Build history of the part. All positions in model axes, mm. Face numbers are marked on the shaded views. A direction names the side the tool comes from. Give positions to 0.01 mm unless a question says otherwise; leave off trailing zeros. Order: outer loops, then holes, each group sorted by start corner. A loop starts at its lowest first (then second) coordinate and runs counter-clockwise, first axis right, second up. Notation, with made-up numbers: M 76.5,4 L 108.5,4 A9 cw 108.5,18 Z; hole C 54,-39.75 d3. An arc over 180 degrees is marked long. One line per item, written item: value.
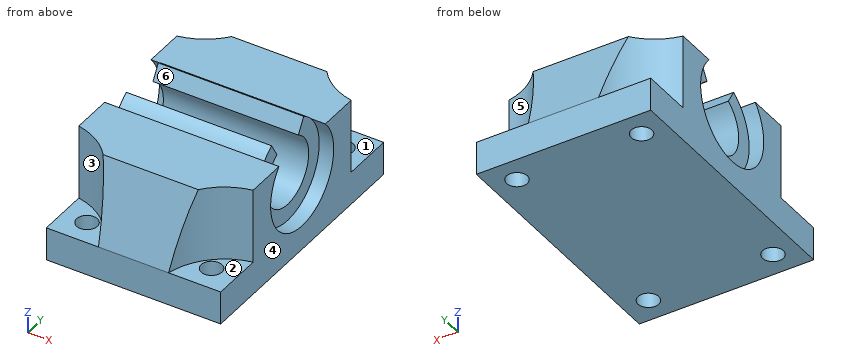
from build123d import *

# Parameters (mm, degrees)
F1_DEPTH = 21
F3_R     = 15.743514377
F4_DEPTH = 33
F5_DEPTH = 17.5
F7_D     = 5


with BuildPart() as f1:
    # F0 (on Right) → F1 (new body, symmetric)
    with BuildSketch(Plane.YZ):
        with BuildLine():
            Line((24.4485357832, 8.14), (8.8170516614, 8.14))
            ThreePointArc((8.8170516614, 8.14), (0, -12), (-8.8170516614, 8.14))
            Line((-8.8170516614, 8.14), (-24.4485357832, 8.14))
            Line((-24.4485357832, 8.14), (-31, -9.86))
            Line((-31, -9.86), (-31, -17.86))
            Line((-31, -17.86), (0, -17.86))
            Line((0, -17.86), (31, -17.86))
            Line((31, -17.86), (31, -9.86))
            Line((31, -9.86), (24.4485357832, 8.14))
        make_face()
    extrude(amount=F1_DEPTH, both=True)

    # F3 (on offset) → F4 (cut)
    with BuildSketch(Plane(origin=(0, 0, -9.86), x_dir=(1, 0, 0), z_dir=(0, 0, -1))):
        with Locations((-23.8725915551, 34.129627049)):
            Circle(F3_R)
        with Locations((-23.8725915551, -34.129627049)):
            Circle(F3_R)
        with Locations((23.8725915551, -34.129627049)):
            Circle(F3_R)
        with Locations((23.8725915551, 34.129627049)):
            Circle(F3_R)
    extrude(amount=-F4_DEPTH, mode=Mode.SUBTRACT)

    # F0 (on Right) → F5 (join, symmetric)
    with BuildSketch(Plane.YZ):
        with BuildLine():
            ThreePointArc((4.0603069037, 6.8930332835), (6.9455905159, 3.9697320294), (8, 0))
            ThreePointArc((8, 0), (-3.9697320294, -6.9455905159), (-4.0603069037, 6.8930332835))
            Line((-4.0603069037, 6.8930332835), (-6.0904603555, 10.3395499253))
            ThreePointArc((-6.0904603555, 10.3395499253), (-7.5344531057, 9.3398081564), (-8.8170516614, 8.14))
            ThreePointArc((-8.8170516614, 8.14), (0, -12), (8.8170516614, 8.14))
            ThreePointArc((8.8170516614, 8.14), (7.5344531057, 9.3398081564), (6.0904603555, 10.3395499253))
            Line((6.0904603555, 10.3395499253), (4.0603069037, 6.8930332835))
        make_face()
    extrude(amount=F5_DEPTH, both=True)

    # F7 (through all)
    with Locations(Plane(origin=(0, 0, -17.86), x_dir=(1, 0, 0), z_dir=(0, 0, -1))):
        with Locations((-15, -25), (-15, 25), (15, 25), (15, -25)):
            Hole(F7_D / 2)


solid = f1.part
1) Saw through at D-D, the plane x = 2. Write the cut outline in (y, z).
Check values:
outline: M -31,-17.86 L 31,-17.86 L 31,-9.86 L 24.45,8.14 L 8.82,8.14 A12 ccw 6.09,10.34 L 4.06,6.89 A8 cw long -4.06,6.89 L -6.09,10.34 A12 ccw -8.82,8.14 L -24.45,8.14 L -31,-9.86 Z
2) Tool access for the marked faces 1, 2 and 3: list every direction of +Z, -Z, +X, -X, +Y, -Y with a clear straight run to the whole face (end or side of a thin tool).
Check values:
face 1: +Z, +X, +Y
face 2: +Z, +X, -Y
face 3: +Z, -X, -Y
3) Saw through at A-A, the plane z = -2.25. Write the cut outline in (x, y).
Check values:
outline: M -21,-18.65 A15.74 cw -9.28,-28.23 L 9.28,-28.23 A15.74 cw 21,-18.65 L 21,-11.79 L 17.5,-11.79 L 17.5,-7.68 L -17.5,-7.68 L -17.5,-11.79 L -21,-11.79 Z; M -21,11.79 L -17.5,11.79 L -17.5,7.68 L 17.5,7.68 L 17.5,11.79 L 21,11.79 L 21,18.65 A15.74 cw 9.28,28.23 L -9.28,28.23 A15.74 cw -21,18.65 Z
4) Drill centre lines: probe 1 along Y at (x, z) = (15, -15); probe 2 along X at (y, z) = (-25, -12.75); probe 3 along Y at (x, z) = (-2.5, -0.25). Where is each one in solid material? Low to high. Write a range as from..to.
Check values:
probe 1: -31..-27.5, -22.5..22.5, 27.5..31
probe 2: -21..-17.5, -12.5..12.5, 17.5..21
probe 3: -27.5..-8, 8..27.5
5) Mould opens along Y. For the marked faces 4, 5 and 6 say: released by +Y, released by -Y, zero draft, split by the parting line, or undercut.
Check values:
face 4: zero draft
face 5: released by +Y
face 6: undercut
6) Saw through at B-B, the plane y = 0. Write the cut outline in (x, z).
Check values:
outline: M -21,-17.86 L 21,-17.86 L 21,-12 L 17.5,-12 L 17.5,-8 L -17.5,-8 L -17.5,-12 L -21,-12 Z
7) Pin check, flat tips, straight feed: pin 1 (8 mm diameter, centred on x = 15, y = -25, fed in from +Z); pin 2 (6 mm diameter, centred on x = -17, y = 26, fed in from +Z); pin 3 (1 mm diameter, centred on y = -23, z = -8, fed in from +X). Stop position of each tip, or through.
Check values:
pin 1: z = 8.14
pin 2: z = -9.86
pin 3: x = 13.26
8) Saw through at C-C, the plane x = 15. Write the cut outline in (y, z), then the cut area to 3 significant figures.
Check values:
outline: M -31,-17.86 L -27.5,-17.86 L -27.5,-9.86 L -31,-9.86 Z; M -22.5,-17.86 L 22.5,-17.86 L 22.5,-9.86 L 21.12,-9.86 L 21.12,8.14 L 8.82,8.14 A12 ccw 6.09,10.34 L 4.06,6.89 A8 cw long -4.06,6.89 L -6.09,10.34 A12 ccw -8.82,8.14 L -21.12,8.14 L -21.12,-9.86 L -22.5,-9.86 Z; M 27.5,-17.86 L 31,-17.86 L 31,-9.86 L 27.5,-9.86 Z
area: 980 mm^2
